Build history of the part. All positions in model axes, mm. A direction names the side the tool comes from. Give positions to 0.01 mm unless a question says otherwise; leave off trailing zeros. Write each loop counter-clockwise with the first axis right and the second up, starting at its lowest first coordinate (ties: lowest second). Pieces come first, ordered by that corner, then holes.
from build123d import *

# Parameters (mm, degrees)
SKETCH1_R           = 32.5
SKETCH1_R_2         = 25
BOSS_EXTRUDE1_DEPTH = 7
SKETCH2_R           = 32
SKETCH2_R_2         = 25.5
CUT_EXTRUDE1_DEPTH  = 0.1
CUT_EXTRUDE2_START  = -0.1
SKETCH3_R           = 32
SKETCH3_R_2         = 25.5
CUT_EXTRUDE2_DEPTH  = 0.1


with BuildPart() as part:
    # Sketch1 → Boss-Extrude1 (new body)
    with BuildSketch(Plane.XY):
        Circle(SKETCH1_R)
        Circle(SKETCH1_R_2, mode=Mode.SUBTRACT)
    extrude(amount=BOSS_EXTRUDE1_DEPTH)

    # Sketch2 → Cut-Extrude1 (cut)
    with BuildSketch(Plane(origin=(0, 0, 0), x_dir=(-1, 0, 0), z_dir=(0, 0, -1))):
        Circle(SKETCH2_R)
        Circle(SKETCH2_R_2, mode=Mode.SUBTRACT)
    extrude(amount=-CUT_EXTRUDE1_DEPTH, mode=Mode.SUBTRACT)

    # Sketch3 → Cut-Extrude2 (cut)
    with BuildSketch(Plane.XY.offset(7).offset(CUT_EXTRUDE2_START)):
        with Locations(Location((0, 0, 0), (0, 0, 180))):
            Circle(SKETCH3_R)
        with Locations(Location((0, 0, 0), (0, 0, 180))):
            Circle(SKETCH3_R_2, mode=Mode.SUBTRACT)
    extrude(amount=CUT_EXTRUDE2_DEPTH, mode=Mode.SUBTRACT)


solid = part.part
(1) 3-axis set-ups, long thin cutter, end or side, ignore diameter. For faces 1 (the face through (21.5, -14.1, 0.1)), 2 (the face through (16.9, -18.8, 7)): which of +Z, -Z, +X, -X, +Y, -Y reach the whole face in a straight line?
(2) Saw through at C-C, the plane z = 2.25. List the corners of the cut face in (x, y).
(3) Mould opens along X. For faces 3 (the face through (21.5, 14.1, 6.9)), 4 (the face through (23.92, -21.52, 7)), 5 (the face through (31, 9.76, 3.45)) say: +X half, -X half, draft (parallel to the pull), parting line (faces both ways), or undercut.
(4) Drop flat-ended pins along their axis: pin 1 (2 mm diameter, centred on x = -10.5, z = 6, fed in from +Y); pin 2 (3 mm diameter, centred on y = -18.5, z = 5, fed in from -X). Give the stop position or say it passes through.
(5) Saw through at A-A, the plane y = 0. List the corners of the cut face in (x, z), plus the area to 3 significant figures.
(6) Saw through at D-D, the plane y = 28. List the corners of the cut face in (x, z), plus the area to 3 significant figures.
(7) Probe line 1 (Y direction, x = 0, z = 2); line 2 (Y direction, x = -6.5, z = 2.25); line 3 (X direction, y = -13, z = 3). List the from-to ranges inside material, lowest first.
Computed values:
1. face 1: -Z
1. face 2: +Z, +X, -X, +Y, -Y
2. outline: circle Ø65 at (0, 0); hole circle Ø50 at (0, 0)
3. face 3: undercut
3. face 4: draft
3. face 5: parting line
4. pin 1: stops at y = 31.08
4. pin 2: stops at x = -27.7
5. outline: (-32.5, 0) - (-32, 0) - (-32, 0.1) - (-25.5, 0.1) - (-25.5, 0) - (-25, 0) - (-25, 7) - (-25.5, 7) - (-25.5, 6.9) - (-32, 6.9) - (-32, 7) - (-32.5, 7) - close; (25, 0) - (25.5, 0) - (25.5, 0.1) - (32, 0.1) - (32, 0) - (32.5, 0) - (32.5, 7) - (32, 7) - (32, 6.9) - (25.5, 6.9) - (25.5, 7) - (25, 7) - close
5. area: 102 mm2
6. outline: (-16.5, 0) - (-15.49, 0) - (-15.49, 0.1) - (15.49, 0.1) - (15.49, 0) - (16.5, 0) - (16.5, 7) - (15.49, 7) - (15.49, 6.9) - (-15.49, 6.9) - (-15.49, 7) - (-16.5, 7) - close
6. area: 225 mm2
7. line 1: y = -32.5 to -25, 25 to 32.5
7. line 2: y = -31.84 to -24.14, 24.14 to 31.84
7. line 3: x = -29.79 to -21.35, 21.35 to 29.79
